from build123d import *

# Parameters (mm, degrees)
ESQUISSE1_W             = 120
ESQUISSE1_H             = 250
BOSS_EXTRU_1_DEPTH      = 6
ESQUISSE2_W             = 15
ESQUISSE2_H             = 6
BOSS_EXTRU_3_DEPTH      = 6
ESQUISSE3_W             = 44.86
ESQUISSE3_H             = 19
ENL_V_MAT_EXTRU_1_DEPTH = 6


with BuildPart() as part:
    # Esquisse1 → Boss.-Extru.1 (new body)
    with BuildSketch(Plane.XY):
        with Locations((-137.920305677, 0)):
            Rectangle(ESQUISSE1_W, ESQUISSE1_H)
    extrude(amount=BOSS_EXTRU_1_DEPTH)

    # Esquisse2 → Boss.-Extru.3 (add)
    with BuildSketch(Plane.XY.offset(6)):
        with Locations((-160.350305677, -128)):
            Rectangle(ESQUISSE2_W, ESQUISSE2_H)
        with Locations((-160.350305677, 128)):
            Rectangle(ESQUISSE2_W, ESQUISSE2_H)
    extrude(amount=-BOSS_EXTRU_3_DEPTH)

    # Esquisse3 → Enlèv. mat.-Extru.1 (cut)
    with BuildSketch(Plane.XY.offset(6)):
        with Locations((-100.350305677, -115.5)):
            Rectangle(ESQUISSE3_W, ESQUISSE3_H)
    extrude(amount=-ENL_V_MAT_EXTRU_1_DEPTH, mode=Mode.SUBTRACT)


solid = part.part
Verification items for the finished model (mm, model axes). A direction names the side the tool comes from. Round coordinates to 2 decimals unless told otherwise and drop trailing zeros. Loops run counter-clockwise (first coordinate to the right, second up) from the corner with the lowest first, then second, coordinate; pieces in that order, holes last. Notation, with made-up numbers: (3, 26) - (56, 26) arc R30 cw to (56, 58) - close; hole circle Ø5 at (40, 70.25). An arc over 180 degrees is marked (long way). Use one line per item in the form item = value.
1. Section check C-C on x = -92.5. Record the cut outline in (y, z), and give its area (3 significant figures).
A:
outline = (-106, 0) - (125, 0) - (125, 6) - (-106, 6) - close
area = 1,390 mm²
2. Section check A-A on z = 1.7. Record the cut outline in (x, y).
A:
outline = (-197.92, -125) - (-167.85, -125) - (-167.85, -131) - (-152.85, -131) - (-152.85, -125) - (-122.78, -125) - (-122.78, -106) - (-77.92, -106) - (-77.92, 125) - (-152.85, 125) - (-152.85, 131) - (-167.85, 131) - (-167.85, 125) - (-197.92, 125) - close
3. Access from +Z, -Z, +X, -X, +Y, -Y to the whole of each face (thin tool, end or side, straight path). Record for faces 1 (the flat face through (-122.78, -116, 3)), 2 (the flat face through (-160, -131, 3)), 3 (the flat face through (-183, -125, 3)), 4 (the flat face through (-152.85, 128, 3)), 5 (the flat face through (-183, 125, 3)).
A:
face_1 = +Z, -Z, +X, -Y
face_2 = +Z, -Z, +X, -X, -Y
face_3 = +Z, -Z, -X, -Y
face_4 = +Z, -Z, +X, +Y
face_5 = +Z, -Z, -X, +Y
4. Gauge pin test, flat ends, axial feed: pin 1 Ø3 at (x, z) = (-141, 1.5) entering from -Y; pin 2 Ø3 at (y, z) = (-111, 4.5) entering from +X; pin 3 Ø3 at (x, y) = (-134.5, 19.5) entering from -Z; pin 4 Ø1.8 at (x, z) = (-187.5, 4) entering from +Y. Record the tip position at first contact, or that the pin passes through.
A:
pin_1 = -125
pin_2 = -122.78
pin_3 = 0
pin_4 = 125
5. Section check B-B on x = -181.5. Record the cut outline in (y, z).
A:
outline = (-125, 0) - (125, 0) - (125, 6) - (-125, 6) - close
6. Scan lines: probe 1 along Y at (x, z) = (-87.5, 2.1); probe 2 along Y at (x, z) = (-142.5, 1.3). Record each from-to range of solid material in increasing order.
A:
probe_1 = -106 to 125
probe_2 = -125 to 125
